Read the model definition and answer for the solid it produces. Units are mm, in the model's axes. A direction names the side the tool comes from. Coordinates: 2 decimals unless noted, no trailing zeros. Write each loop counter-clockwise with the first axis right and the second up, starting at its lowest first coordinate (ties: lowest second). Pieces come first, ordered by that corner, then holes. Notation, with made-up numbers: (51.25, 49.5) - (107.25, 49.5) arc R9 cw to (107.25, 64.5) - close; hole circle Ø10 at (89.25, 71). An arc over 180 degrees is marked (long way). Use a Markdown table: item, result.
from build123d import *

# Parameters (mm, degrees)
EXTRUDE_1_DEPTH              = 5
HOLE_WIZARD_M8_2_AT_2_COUNT  = 2
HOLE_WIZARD_M8_2_AT_2_PITCH  = 140
HOLE_WIZARD_M8_2_AT_3_COUNT  = 2
HOLE_WIZARD_M8_2_AT_3_PITCH  = 169.189243157
HOLE_WIZARD_M8_2_AT_4_COUNT  = 2
HOLE_WIZARD_M8_2_AT_4_PITCH  = 95
SKETCH_10_W                  = 5
SKETCH_10_H                  = 45
EXTRUDE_2_DEPTH              = 260
FILLET_1_R                   = 5
CUT_EXTRUDE_5_DEPTH          = 344.547667726
HOLE_WIZARD_M5_1_D           = 5.5
HOLE_WIZARD_M5_1_CBORE_D     = 11
HOLE_WIZARD_M5_1_CBORE_DEPTH = 0.5


with BuildPart() as part:
    # 草图1 → 凸台-拉伸1 (new body)
    with BuildSketch(Plane(origin=(0, 0, 0), x_dir=(1, 0, 0), z_dir=(0, 1, 0))):
        Polygon((0, 0), (0, -260), (210, -260), (210, 0), (170, 0), (170, -80), (40, -80), (40, 0), align=None)
    extrude(amount=EXTRUDE_1_DEPTH)

    # 草图9 → M8 内六角花形沉头螺钉的锥形沉头孔2 (revolve, cut)
    with BuildSketch(Plane(origin=(57.5, 5, 230), x_dir=(0, 0, 1), z_dir=(1, 0, 0))):
        Polygon((0, 0), (0, 5), (4.5, 5), (4.5, 4.3), (8.8, 0), align=None)
    hole_wizard_m8_2 = revolve(axis=Axis((57.5, 11.35, 230), (0, -1, 0)), mode=Mode.SUBTRACT)

    # M8 内六角花形沉头螺钉的锥形沉头孔2 at 2: M8 内六角花形沉头螺钉的锥形沉头孔2 ×2
    with Locations(*[(0, 0, -i * HOLE_WIZARD_M8_2_AT_2_PITCH) for i in range(1, HOLE_WIZARD_M8_2_AT_2_COUNT)]):
        add(hole_wizard_m8_2, mode=Mode.SUBTRACT)

    # M8 内六角花形沉头螺钉的锥形沉头孔2 at 3: M8 内六角花形沉头螺钉的锥形沉头孔2 ×2
    with Locations(*[Vector(0.5615014183372644, 0, -0.8274757743917585) * (i * HOLE_WIZARD_M8_2_AT_3_PITCH) for i in range(1, HOLE_WIZARD_M8_2_AT_3_COUNT)]):
        add(hole_wizard_m8_2, mode=Mode.SUBTRACT)

    # M8 内六角花形沉头螺钉的锥形沉头孔2 at 4: M8 内六角花形沉头螺钉的锥形沉头孔2 ×2
    with Locations(*[(i * HOLE_WIZARD_M8_2_AT_4_PITCH, 0, 0) for i in range(1, HOLE_WIZARD_M8_2_AT_4_COUNT)]):
        add(hole_wizard_m8_2, mode=Mode.SUBTRACT)

    # 草图10 → 凸台-拉伸2 (add, through all)
    with BuildSketch(Plane(origin=(0, 0, 0), x_dir=(-1, 0, 0), z_dir=(0, 0, -1))):
        with Locations((2.5, 22.5)):
            Rectangle(SKETCH_10_W, SKETCH_10_H)
        with Locations((-212.5, 22.5)):
            Rectangle(SKETCH_10_W, SKETCH_10_H)
    extrude(amount=-EXTRUDE_2_DEPTH)

    # 圆角1
    fillet_1_edges = [part.edges().sort_by_distance(p)[0] for p in [
        (-5, 0, 130),
        (215, 0, 130),
    ]]
    fillet(fillet_1_edges, radius=FILLET_1_R)

    # 草图11 → 切除-拉伸5 (cut, through all)
    with BuildSketch(Plane(origin=(215, 0, 0), x_dir=(0, 0, -1), z_dir=(1, 0, 0))):
        with BuildLine():
            Line((-15, 29), (-30, 29))
            ThreePointArc((-30, 29), (-34, 25), (-30, 21))
            Line((-30, 21), (-15, 21))
            ThreePointArc((-15, 21), (-11, 25), (-15, 29))
        make_face()
        with BuildLine():
            Line((-230, 21), (-245, 21))
            ThreePointArc((-245, 21), (-249, 25), (-245, 29))
            Line((-245, 29), (-230, 29))
            ThreePointArc((-230, 29), (-226, 25), (-230, 21))
        make_face()
    extrude(amount=-CUT_EXTRUDE_5_DEPTH, mode=Mode.SUBTRACT)

    # M5 六角头螺栓的柱形沉头孔1 (through all)
    with Locations(Plane(origin=(0, 5, 0), x_dir=(1, 0, 0), z_dir=(0, 1, 0))):
        with Locations((176.25, -129.5), (8, -86), (41.25, -255.25)):
            CounterBoreHole(HOLE_WIZARD_M5_1_D / 2, HOLE_WIZARD_M5_1_CBORE_D / 2, HOLE_WIZARD_M5_1_CBORE_DEPTH)


solid = part.part
(1) For faces 1 (the flat face through (0, 25, 128)), 2 (the flat face through (179, 4.5, 132)), 3 (the cylindrical face through (59.22, 0.35, 234.16)), determine the directions among +Z, -Z, +X, -X, +Y, -Y from which every point of the face is accessible in a straight line to the end or side of a thin tool.
Report:
| item | result |
|---|---|
| face 1 | +Z, -Z, +Y |
| face 2 | +Y |
| face 3 | +Y, -Y |
(2) A cutting plane is placed at C-C, the plane z = 60. Write down the section's boundary in (x, y).
Report:
| item | result |
|---|---|
| outline | (-5, 5) arc R5 ccw to (0, 0) - (40, 0) - (40, 5) - (0, 5) - (0, 45) - (-5, 45) - close; (170, 0) - (210, 0) arc R5 ccw to (215, 5) - (215, 45) - (210, 45) - (210, 5) - (170, 5) - close |
(3) The mould has two halves that part along X. Classify faces 4 (the flat face through (210, 25, 128)), 5 (the flat face through (106, 0, 157)): pulls with the +X half, pulls with the -X half, needs draft (parallel to the pull), parting line crosses it, or undercut.
Report:
| item | result |
|---|---|
| face 4 | undercut |
| face 5 | needs draft |
(4) A cutting plane is placed at D-D, the plane x = 57.5. Write down the section's boundary in (y, z), and give its area (3 significant figures).
Report:
| item | result |
|---|---|
| outline | (0, 80) - (5, 80) - (5, 81.2) - (0.7, 85.5) - (0, 85.5) - close; (0, 94.5) - (0.7, 94.5) - (5, 98.8) - (5, 221.2) - (0.7, 225.5) - (0, 225.5) - close; (0, 234.5) - (0.7, 234.5) - (5, 238.8) - (5, 260) - (0, 260) - close |
| area | 773 mm² |
(5) A cutting plane is placed at A-A, the plane x = 8. Write down the section's boundary in (y, z).
Report:
| item | result |
|---|---|
| outline | (0, 0) - (5, 0) - (5, 80.5) - (4.5, 80.5) - (4.5, 83.25) - (0, 83.25) - close; (0, 88.75) - (4.5, 88.75) - (4.5, 91.5) - (5, 91.5) - (5, 260) - (0, 260) - close |
(6) A cutting plane is placed at B-B, the plane y = 14.5. Write down the section's boundary in (x, z).
Report:
| item | result |
|---|---|
| outline | (-5, 0) - (0, 0) - (0, 260) - (-5, 260) - close; (210, 0) - (215, 0) - (215, 260) - (210, 260) - close |
(7) Straight lines are drawn through the part: L1, parallel to Z at x = 176, y = 3; L2, parallel to X at y = 17, z = 55; L3, parallel to Z at x = 57.5, y = 0.2. For each, find the intervals that lie inside material, in ascending order.
Report:
| item | result |
|---|---|
| L1 | z = 0 to 126.76, 132.24 to 260 |
| L2 | x = -5 to 0, 210 to 215 |
| L3 | z = 80 to 85.5, 94.5 to 225.5, 234.5 to 260 |
(8) Each of these flat-tipped pins is pushed along its axis until it touches: P1, Ø1.5, axis at x = -1.5, z = 237.5, coming from the -Y side; P2, Ø10, axis at x = 158.5, z = 167, coming from the +Y side; P3, Ø9, axis at x = 177, z = 130, coming from the +Y side. Where does it stop, or does it pass through?
Report:
| item | result |
|---|---|
| P1 | stops at y = 0.06 |
| P2 | stops at y = 5 |
| P3 | stops at y = 4.5 |
